Check sheet for the modelled part. Datum: model origin and axes. Units: mm. A direction names the side the tool comes from. Coordinates: 2 decimals unless noted, no trailing zeros. Loops run counter-clockwise (first coordinate to the right, second up) from the corner with the lowest first, then second, coordinate; pieces in that order, holes last.
```python
from build123d import *

# Parameters (mm, degrees)
F0_R            = 11
F1_DEPTH        = 4.2
F3_DEPTH        = 4.201
F3_COPIES_COUNT = 12
F5_R            = 3.2
F6_DEPTH        = 3
F7_W            = 3.6
F7_H            = 3.6
F8_DEPTH        = 7.201


# Not quite as in the source:
# - a pattern or mirror of a feature is missing from the dataset's text; its kind, count and spacing are read off the source's solid


with BuildPart() as f1:
    # F0 (on Top) → F1 (new body)
    with BuildSketch(Plane.XY):
        Circle(F0_R)
    extrude(amount=F1_DEPTH)

    # F2 (on face) → F3 (cut, through all)
    with BuildSketch(Plane(origin=(0, 0, 0), x_dir=(1, 0, 0), z_dir=(0, 0, -1))):
        with BuildLine():
            ThreePointArc((6.9957357891, 0.2442964769), (6.9989338661, 0.1221668451), (7, 0))
            Line((7, 0), (8.3441911265, 0))
            Line((8.3441911265, 0), (11, 0))
            ThreePointArc((11, 0), (10.9292904124, 1.2452353514), (10.7180707126, 2.4744615978))
            Line((10.7180707126, 2.4744615978), (6.9957357891, 0.2442964769))
        make_face()
        with BuildLine():
            Line((8.3441911265, 0), (7, 0))
            Line((7, 0), (6.9957357891, -0.2442964769))
            Line((6.9957357891, -0.2442964769), (10.7180707126, -2.4744615978))
            ThreePointArc((10.7180707126, -2.4744615978), (10.9292904124, -1.2452353514), (11, 0))
            Line((11, 0), (8.3441911265, 0))
        make_face()
    f3 = extrude(amount=-F3_DEPTH, mode=Mode.SUBTRACT)

    # F3_copies: F3 ×12 about axis
    f3_copies_axis = Axis((0, 0, 0), (0, 0, 1))
    for i in range(1, F3_COPIES_COUNT):
        add(f3.rotate(f3_copies_axis, i * 360 / F3_COPIES_COUNT), mode=Mode.SUBTRACT)

    # F5 (on face) → F6 (join)
    with BuildSketch(Plane(origin=(0, 0, 0), x_dir=(1, 0, 0), z_dir=(0, 0, -1))):
        with Locations((-0.0057600341, -0.0028142263)):
            Circle(F5_R)
    extrude(amount=F6_DEPTH)

    # F7 (on face) → F8 (cut, through all)
    with BuildSketch(Plane(origin=(0, 0, -3), x_dir=(1, 0, 0), z_dir=(0, 0, -1))):
        with Locations((0.0985847846, 0.0223461993)):
            Rectangle(F7_W, F7_H)
    extrude(amount=-F8_DEPTH, mode=Mode.SUBTRACT)


solid = f1.part
```
1) Section check D-D on y = 8.5. Enter the section's corners in (x, z), plus the area to 3 significant figures.
Answer sheet:
outline: (-3.25, 0) - (-1.15, 0) - (-1.15, 4.2) - (-3.25, 4.2) - close; (1.15, 0) - (3.25, 0) - (3.25, 4.2) - (1.15, 4.2) - close
area: 17.7 mm2
2) Section check B-B on x = -0.75. Enter the section's corners in (y, z).
Answer sheet:
outline: (-7.84, 0) - (-3.11, 0) - (-3.11, -3) - (-1.82, -3) - (-1.82, 4.2) - (-7.84, 4.2) - close; (1.78, -3) - (3.12, -3) - (3.12, 0) - (7.84, 0) - (7.84, 4.2) - (1.78, 4.2) - close
3) Section check C-C on z = -2.5. Enter the section's corners in (x, y).
Answer sheet:
outline: circle Ø6.4 at (-0.01, 0); hole (-1.7, -1.82) - (1.9, -1.82) - (1.9, 1.78) - (-1.7, 1.78) - close
4) Mould release check, pull along X, two halves, no side actions. Record for faces 1 (the flat face through (1.344, -8.831, 2.071)), 2 (the flat face through (1.375, 8.883, 2.071)), 3 (the flat face through (-8.883, 1.375, 2.071)), 4 (the flat face through (0, -2, 4.2)): +X half, -X half, draft (parallel to the pull), parting line (faces both ways), or undercut.
Answer sheet:
face 1: undercut
face 2: undercut
face 3: -X half
face 4: draft
5) Scan lines: line 1 (Z direction, x = -3, y = -7.75); line 2 (Y direction, x = 0.25, z = -1); line 3 (X direction, y = -8.75, z = 1.25). Record each from-to range of solid material in increasing order.
Answer sheet:
line 1: z = 0 to 4.2
line 2: y = -3.19 to -1.82, 1.78 to 3.19
line 3: x = -3.24 to -1.3, 1.3 to 3.24
6) Set-up check for faces 5 (the flat face through (6.976, 5.579, 2.071)), 6 (the flat face through (-1.375, -8.883, 2.071)), 7 (the flat face through (-8.831, -1.344, 2.071)), 8 (the flat face through (0, -1.822, 1)), 9 (the flat face through (-1.344, 8.831, 2.071)): record each of +Z, -Z, +X, -X, +Y, -Y from which the full face is reachable in a straight line by a thin tool's end or side.
Answer sheet:
face 5: +Z, -Z, +X
face 6: +Z, -Z, -Y
face 7: +Z, -Z, -X
face 8: +Z, -Z
face 9: +Z, -Z, +Y
7) Depth check by flat-ended pin: pin 1 (1.1 mm diameter, centred on x = 0.5, z = 0.5, fed in from +Y); pin 2 (1 mm diameter, centred on y = 5, z = 3, fed in from +X); pin 3 (3 mm diameter, centred on y = 0, z = 1.5, fed in from +X). Enter the tip coordinate at first touch or a pass-through.
Answer sheet:
pin 1: stops at y = 8.34
pin 2: stops at x = 6.93
pin 3: stops at x = 9.09
8) Section check A-A on y = -0.5. Enter the section's corners in (x, z), plus the area to 3 significant figures.
Answer sheet:
outline: (-7.42, 0) - (-3.17, 0) - (-3.17, -3) - (-1.7, -3) - (-1.7, 4.2) - (-7.42, 4.2) - close; (1.9, -3) - (3.15, -3) - (3.15, 0) - (7.42, 0) - (7.42, 4.2) - (1.9, 4.2) - close
area: 55.4 mm2
